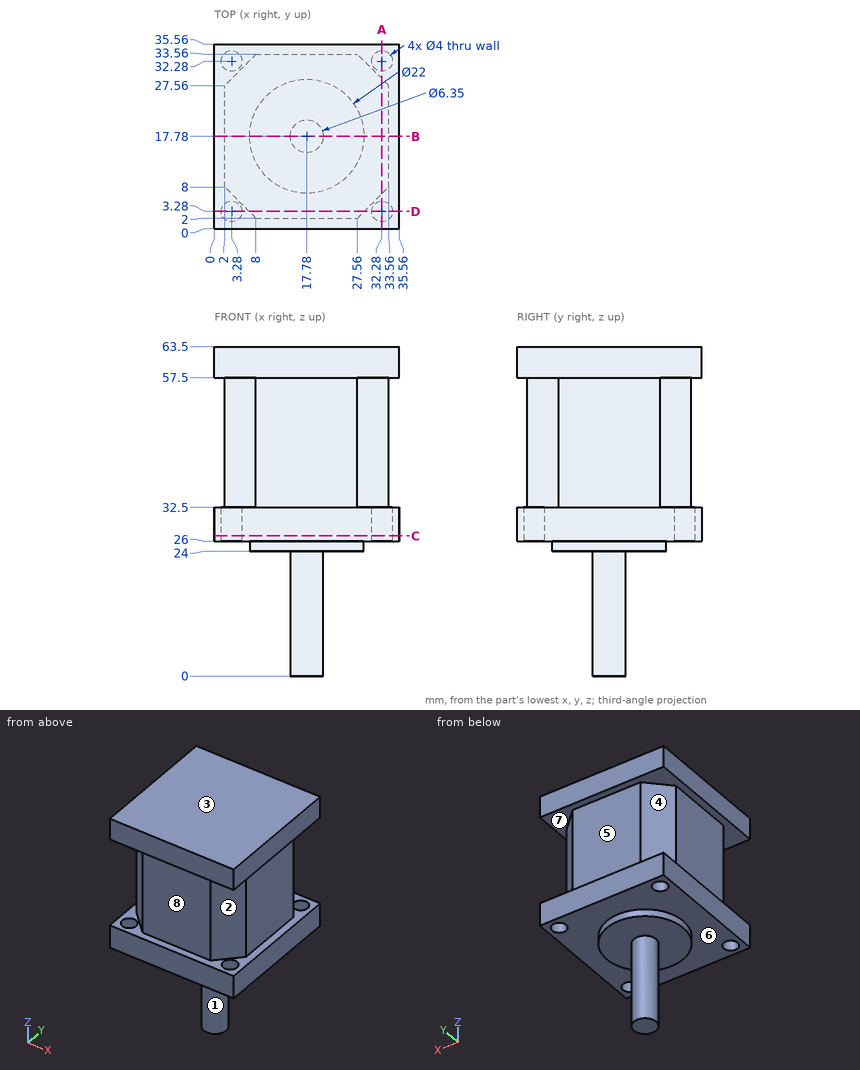
Input: dimensioned drawing with shaded views. Units: mm. Origin: part minimum x, y, z. A direction names the side the tool comes from. Give positions to 0.01 mm unless a question says otherwise; leave off trailing zeros. Order: outer loops, then holes, each group sorted by start corner. A loop starts at its lowest first (then second) coordinate and runs counter-clockwise, first axis right, second up. Notation, with made-up numbers: (81.5, 46) -> (91.5, 46) arc R30 ccw to (91.5, 81) -> close; hole circle Ø9 at (-35, 25). An arc over 180 degrees is marked (long way). Answer as a JSON object with one key per item and string values.
Q1. Material intervals for probe 1 along Y at (x, z) = (32.28, 28.5); probe 2 along Y at (x, z) = (31.5, 29.5); probe 3 along X at (y, z) = (32, 31), sorted ascending.
Entries:
{"probe 1": "y = 0 to 1.28, 5.28 to 30.28, 34.28 to 35.56", "probe 2": "y = 0 to 1.44, 5.12 to 30.44, 34.12 to 35.56", "probe 3": "x = 0 to 1.3, 5.26 to 30.3, 34.26 to 35.56"}
Q2. Section A-A (x = 32.28). Output: boundary loops of the cut face in (y, z).
Entries:
{"outline": "(0, 26) -> (1.28, 26) -> (1.28, 32.5) -> (0, 32.5) -> close; (0, 57.5) -> (6.72, 57.5) -> (6.72, 32.5) -> (5.28, 32.5) -> (5.28, 26) -> (30.28, 26) -> (30.28, 32.5) -> (28.84, 32.5) -> (28.84, 57.5) -> (35.56, 57.5) -> (35.56, 63.5) -> (0, 63.5) -> close; (34.28, 26) -> (35.56, 26) -> (35.56, 32.5) -> (34.28, 32.5) -> close"}
Q3. Access query for the marked faces 4, 5, 6, 7 and 8. Directions: +Z, -Z, +X, -X, +Y, -Y. A direction counts if a zero-diameter tool reaches every point of the face in a straight line with its end or side. Return the directions, or none.
Entries:
{"face 4": "-X, +Y", "face 5": "+X, -X, +Y", "face 6": "-Z", "face 7": "none", "face 8": "+X, -X, -Y"}
Q4. Section C-C (z = 27). Output: boundary loops of the cut face in (x, y).
Entries:
{"outline": "(0, 0) -> (35.56, 0) -> (35.56, 35.56) -> (0, 35.56) -> close; hole circle Ø4 at (3.28, 3.28); hole circle Ø4 at (3.28, 32.28); hole circle Ø4 at (32.28, 3.28); hole circle Ø4 at (32.28, 32.28)"}
Q5. Section B-B (y = 17.78). Output: boundary loops of the cut face in (x, z) (3 decimals).
Entries:
{"outline": "(0, 26) -> (6.78, 26) -> (6.78, 24) -> (14.605, 24) -> (14.605, 0) -> (20.955, 0) -> (20.955, 24) -> (28.78, 24) -> (28.78, 26) -> (35.56, 26) -> (35.56, 32.5) -> (33.56, 32.5) -> (33.56, 57.5) -> (35.56, 57.5) -> (35.56, 63.5) -> (0, 63.5) -> (0, 57.5) -> (2, 57.5) -> (2, 32.5) -> (0, 32.5) -> close"}
Q6. First-contact query: pin 1 (15.5 mm diameter, centred on x = 22, z = 40.5, fed in from -Y); pin 2 (5 mm diameter, centred on x = 32.28, y = 32.28, fed in from -Z); pin 3 (15.5 mm diameter, centred on x = 22, z = 41, fed in from +Y). Flat tips, straight axial feed; report the tip coordinate or a pass-through.
Entries:
{"pin 1": "stops at y = 2", "pin 2": "stops at z = 26", "pin 3": "stops at y = 33.56"}
Q7. Draft query along Z for the marked faces 1, 2 and 3. Return one class per face: released by +Z, released by -Z, zero draft, split by the parting line, or undercut.
Entries:
{"face 1": "zero draft", "face 2": "undercut", "face 3": "released by +Z"}
